Autodesk Inventor part; units mm, degrees
ref_plane "YZ Plane" through (0, 0, 0) normal (1, 0, 0) x (0, 1, 0)
ref_plane "XZ Plane" through (0, 0, 0) normal (0, 1, 0) x (-1, 0, 0)
ref_plane "XY Plane" through (0, 0, 0) normal (0, 0, 1) x (1, 0, 0)
sketch "Sketch1" plane through (0, 0, 0) normal (0, 0, 1) x (1, 0, 0)
  circle A0 centre (0, 0) radius 60.325
  circle A1 centre (0, 0) radius 47.625
  dimension "d0" = 120.65
  dimension "d1" = 12.7
extrude "Extrusion1" add sketch "Sketch1" against normal blind 9.525
sketch "Sketch2" plane through (0, 0, 0) normal (0, 0, 1) x (1, 0, 0)
  circle A0 centre (0, 0) radius 50.8
  circle A1 centre (0, 0) radius 47.625
  dimension "d4" = 101.6
extrude "Extrusion2" cut sketch "Sketch2" against normal blind 6.35 contours A0 | A1
sketch "Sketch3" plane through (0, 0, 0) normal (0, 0, 1) x (1, 0, 0)
  circle A0 centre (0, 0) radius 53.848 construction
  circle A1 centre (0, 0) radius 60.325
  point P0 (0, 53.848)
  point P1 (-53.848, 0)
  point P2 (0, -53.848)
  point P3 (53.848, 0)
  dimension "d7" = 53.848
  dimension "d10" = 360
hole "Hole1" at (0, 53.848, 0) at (-53.848, 0, 0) at (0, -53.848, 0) at (53.848, 0, 0) direction (0, 0, -1) diameter 3.9624 end through all
sketch "Sketch4" plane through (0, 0, -9.525) normal (0, 0, -1) x (-1, 0, 0)
  circle A0 centre (0, 0) radius 47.9425
  circle A1 centre (0, 0) radius 47.625
  dimension "d19" = 95.885
extrude "Extrusion3" cut sketch "Sketch4" against normal blind 6.35
sketch "Sketch5" plane through (0, 0, 0) normal (0, 0, 1) x (1, 0, 0)
  circle A0 centre (0, 0) radius 55.5625 construction
  line L0 (0, 0) -> (0, 55.5625) construction
  circle A1 centre (0, 0) radius 60.325 construction
  line L1 (-60.325, 0) -> (60.325, 0) construction
  line L2 (-19.05, -52.1947) -> (-19.05, 52.1947) construction
  line L3 (19.05, -52.1947) -> (19.05, 52.1947) construction
  dimension "d22" = 111.125
  dimension "d25" = 19.05
  dimension "d26" = 19.05
  dimension "d47" = 104.394
hole "Hole2" at (-19.05, 52.1947, 0) at (19.05, 52.1947, 0) at (-19.05, -52.1947, 0) at (19.05, -52.1947, 0) direction (0, 0, -1) diameter 3.9624 end through all
sketch "Sketch6" plane through (0, 0, 0) normal (0, 0, 1) x (1, 0, 0)
  circle A0 centre (0, 0) radius 55.5625 construction
  line L0 (0, 0) -> (-39.2886, 39.2886) construction
  line L1 (0, 0) -> (-60.7712, 0) construction
  point P0 (-39.2886, -39.2886)
  point P1 (39.2886, -39.2886)
  point P2 (39.2886, 39.2886)
  dimension "d34" = 111.125
  dimension "d35" = 45
  dimension "d38" = 360
hole "Hole3" at (-39.2886, 39.2886, 0) at (-39.2886, -39.2886, 0) at (39.2886, -39.2886, 0) at (39.2886, 39.2886, 0) direction (0, 0, -1) diameter 4.9784 end through all
sketch "Sketch7" plane through (0, 0, 0) normal (0, 0, 1) x (1, 0, 0)
  circle A0 centre (0, 0) radius 54.61 construction
  line L0 (0, 0) -> (0, 54.61) construction
  line L1 (0, 0) -> (7.6002, 54.0785) construction
  circle A1 centre (0, 0) radius 60.325 construction
  line L2 (-60.325, 0) -> (60.325, 0) construction
  circle A2 centre (39.2886, -39.2886) radius 2.4892
  circle A3 centre (-39.2886, 39.2886) radius 2.4892
  circle A4 centre (-39.2886, -39.2886) radius 2.4892
  circle A5 centre (39.2886, 39.2886) radius 2.4892
  circle A6 centre (-19.05, -52.1947) radius 1.9812
  circle A7 centre (-19.05, 52.1947) radius 1.9812
  circle A8 centre (19.05, 52.1947) radius 1.9812
  circle A9 centre (19.05, -52.1947) radius 1.9812
  circle A10 centre (0, -53.848) radius 1.9812
  circle A11 centre (0, 53.848) radius 1.9812
  circle A12 centre (-53.848, 0) radius 1.9812
  circle A13 centre (53.848, 0) radius 1.9812
  circle A14 centre (0, 0) radius 50.8
  circle A15 centre (0, 0) radius 60.325
  point P0 (7.6002, -54.0785)
  dimension "d49" = 109.22
  dimension "d50" = 8
hole "Hole4" at (7.6002, 54.0785, 0) at (7.6002, -54.0785, 0) direction (0, 0, -1) diameter 6.35 end through all
properties part number "LS-001" material "Aluminum 6061"
Design review of the part built by this model. Coordinates are the model's own, in mm. A direction names the side the tool comes from. Coordinates: 2 decimals unless noted, no trailing zeros. Order: outer loops, then holes, each group sorted by start corner. A loop starts at its lowest first (then second) coordinate and runs counter-clockwise, first axis right, second up. Notation, with made-up numbers: (77.25, 57) - (129.25, 57) arc R13 ccw to (129.25, 70) - close; hole circle Ø6 at (14, -33). An arc over 180 degrees is marked (long way). Put each result on its own line as item: value.
1) Take a section at C-C, the plane x = 24. Give the boundary of the cut face in (y, z) (3 decimals).
Response values:
outline: (-55.345, -9.525) - (-41.503, -9.525) - (-41.503, -6.35) - (-44.773, -6.35) - (-44.773, 0) - (-55.345, 0) - close; (41.503, -9.525) - (55.345, -9.525) - (55.345, 0) - (44.773, 0) - (44.773, -6.35) - (41.503, -6.35) - close
2) Wall thickness on L1, parallel to Y at x = 0, z = -4 (3 decimals); L2, parallel to Y at x = 19.05, z = -4; L3, parallel to Y at x = -28, z = -3.75: over which ranges is each line inside the solid? List them lowest first. Write a range as from..to.
Response values:
L1: y = -60.325..-55.829, -51.867..-50.8, 50.8..51.867, 55.829..60.325
L2: y = -57.24..-54.18, -50.21..-47.09, 47.09..50.21, 54.18..57.24
L3: y = -53.43..-42.39, 42.39..53.43
3) The part is to be moulded in two halves that separate along X. For faces 1 (the face through (39.2, -36.8, -4.8)), 2 (the face through (18, 45, -9.525)), 3 (the face through (-60.267, 2.652, -4.696)), say which applies: released by +X, released by -X, zero draft, split by the parting line, or undercut.
Response values:
face 1: undercut
face 2: zero draft
face 3: split by the parting line
4) Tool access review of faces 4 (the face through (-11.012, -49.592, -3.131)), 5 (the face through (-37.774, -37.313, -4.829)): name each direction out of +Z, -Z, +X, -X, +Y, -Y from which nothing blocks a thin tool from reaching the whole face with its end or side.
Response values:
face 4: +Z
face 5: +Z, -Z
5) Take a section at A-A, the plane x = 0. Count the separate pieces of the cut face and the enclosed holes in it, and give its area (3 significant figures).
Response values:
separate pieces: 4
enclosed holes: 0
area: 124 mm²
6) Insertion check: P1, Ø3, axis at x = -37.5, z = -8, coming from the +Y side; P2, Ø1.5, axis at y = 32.5, z = -7.5, coming from the +X side; P3, Ø1, axis at x = 10.5, z = -1, coming from the +Y side. Each pin has a flat end and moves straight along its axis. Give the tip position at first contact, or say it passes through.
Response values:
P1: stops at y = 48.41
P2: stops at x = 51.29
P3: stops at y = 59.49
